```python
from build123d import *

# Parameters (mm, degrees)
F1_DEPTH = 25.4


with BuildPart() as f1:
    # F0 (on Front) → F1 (new body)
    with BuildSketch(Plane.XZ):
        with BuildLine():
            Line((6.35, -17.78), (6.35, -10.992656))
            ThreePointArc((6.35, -10.992656), (0, 12.69492), (-6.35, -10.992656))
            Line((-6.35, -10.992656), (-6.35, -17.78))
            Line((-6.35, -17.78), (-13.745875, -38.1))
            Line((-13.745875, -38.1), (-26.9875, -38.1))
            Line((-26.9875, -38.1), (-26.9875, -44.45))
            Line((-26.9875, -44.45), (26.9875, -44.45))
            Line((26.9875, -44.45), (26.9875, -38.1))
            Line((26.9875, -38.1), (13.745875, -38.1))
            Line((13.745875, -38.1), (6.35, -17.78))
        make_face()
    extrude(amount=F1_DEPTH)


solid = f1.part
```
Geometry: final body of the model. Coordinates: model frame, mm. A direction names the side the tool comes from. Round coordinates to 2 decimals unless told otherwise and drop trailing zeros. Write each loop counter-clockwise with the first axis right and the second up, starting at its lowest first coordinate (ties: lowest second). Pieces come first, ordered by that corner, then holes.
Item 1: Section query A-A (x = 8). Return loops of the section in (y, z), plus the area to 3 significant figures.
Item 2: Set-up query: faces 1 (the face through (-9.996, -12.522, -27.798)), 2 (the face through (-20, -13, -38.1)), 3 (the face through (6.35, -13, -14)), 4 (the face through (20, -13, -38.1)). Return all of +Z, -Z, +X, -X, +Y, -Y with unobstructed straight access to the full face (end or side cutting, diameter ignored); none if empty.
Item 3: Section query D-D (x = -21). Return loops of the section in (y, z), plus the area to 3 significant figures.
Item 4: Section query C-C (z = 0). Return loops of the section in (x, y), plus the area to 3 significant figures.
Item 5: Pin query (flat end, axial travel): P1, Ø8, axis at x = -5.5, y = -11, coming from the +Z side; P2, Ø8, axis at y = -4, z = -8, coming from the +X side; P3, Ø10.5, axis at x = 20, y = -18.5, coming from the +Z side; P4, Ø5, axis at x = -12, z = -19.5, coming from the +Y side. Return the tip coordinate at first contact, or that it passes through.
Item 6: Section query B-B (y = -14.25). Return loops of the section in (x, z), plus the area to 3 significant figures.
Item 7: Material intervals for L1, parallel to X at y = -8.75, z = -14.5; L2, parallel to Z at x = -25, y = -10.75, sorted ascending.
Completed:
1. outline: (-25.4, -44.45) - (0, -44.45) - (0, -22.31) - (-25.4, -22.31) - close; (-25.4, -9.86) - (0, -9.86) - (0, 9.86) - (-25.4, 9.86) - close
1. area: 1,060 mm2
2. face 1: -X, +Y, -Y
2. face 2: +Z, -X, +Y, -Y
2. face 3: +X, +Y, -Y
2. face 4: +Z, +X, +Y, -Y
3. outline: (-25.4, -44.45) - (0, -44.45) - (0, -38.1) - (-25.4, -38.1) - close
3. area: 161 mm2
4. outline: (-12.69, -25.4) - (12.69, -25.4) - (12.69, 0) - (-12.69, 0) - close
4. area: 645 mm2
5. P1: stops at z = 12.61
5. P2: stops at x = 12.05
5. P3: stops at z = -38.1
5. P4: passes through
6. outline: (-26.99, -44.45) - (26.99, -44.45) - (26.99, -38.1) - (13.75, -38.1) - (6.35, -17.78) - (6.35, -10.99) arc R12.69 ccw (long way) to (-6.35, -10.99) - (-6.35, -17.78) - (-13.75, -38.1) - (-26.99, -38.1) - close
6. area: 1,330 mm2
7. L1: x = -6.35 to 6.35
7. L2: z = -44.45 to -38.1
